from build123d import *
from build123d.topology import SkipClean

# Parameters (mm, degrees)
SKETCH1_W           = 30
SKETCH1_H           = 30
SKETCH1_W_2         = 2
SKETCH1_H_2         = 10
BOSS_EXTRUDE1_DEPTH = 75
SKETCH2_W           = 30
SKETCH2_H           = 22.5
CUT_EXTRUDE1_DEPTH  = 75
SKETCH3_W           = 26
SKETCH3_H           = 30.082215134
CUT_EXTRUDE2_DEPTH  = 28
SKETCH5_R           = 2.5
CUT_EXTRUDE3_DEPTH  = 38
BOSS_EXTRUDE2_DEPTH = 2
BOSS_EXTRUDE3_START = 2
BOSS_EXTRUDE3_DEPTH = 2
SKETCH9_R           = 2.5
CUT_EXTRUDE4_DEPTH  = 169.967145294


with BuildPart() as part:
    # Sketch1 → Boss-Extrude1 (new body)
    with BuildSketch(Plane.XY):
        Rectangle(SKETCH1_W, SKETCH1_H)
        with BuildLine():
            Line((50.917737084, -85.641756384), (53, -85.641756384))
            ThreePointArc((53, -85.641756384), (42.989370072, -49.687860894), (15, -25))
            Line((15, -25), (14.157929479, -26.814088542))
            ThreePointArc((14.157929479, -26.814088542), (41.246515654, -50.786104008), (50.917737084, -85.641756384))
        make_face()
        with Locations((14, -20)):
            Rectangle(SKETCH1_W_2, SKETCH1_H_2)
        Polygon((14.157929479, -26.814088542), (15, -25), (13, -25), (13, -26.814088542), align=None)
        with BuildLine():
            Line((12.135037198, -143.180046466), (13, -144.983332176))
            ThreePointArc((13, -144.983332176), (41.796634815, -121.242036174), (53, -85.641756384))
            Line((53, -85.641756384), (50.917737084, -85.641756384))
            ThreePointArc((50.917737084, -85.641756384), (40.047121172, -120.154156399), (12.135037198, -143.180046466))
        make_face()
    extrude(amount=BOSS_EXTRUDE1_DEPTH)

    # Sketch2 → Cut-Extrude1 (cut)
    with BuildSketch(Plane(origin=(0, 15, 0), x_dir=(1, 0, 0), z_dir=(0, 1, 0))):
        with Locations((0, -11.25)):
            Rectangle(SKETCH2_W, SKETCH2_H)
        with Locations((0, -63.75)):
            Rectangle(SKETCH2_W, SKETCH2_H)
    extrude(amount=-CUT_EXTRUDE1_DEPTH, mode=Mode.SUBTRACT)

    # Sketch3 → Cut-Extrude2 (cut)
    with BuildSketch(Plane.ZY.offset(15)):
        with Locations((37.5, 0.030332794)):
            Rectangle(SKETCH3_W, SKETCH3_H)
    extrude(amount=-CUT_EXTRUDE2_DEPTH, mode=Mode.SUBTRACT)

    # Sketch5 → Cut-Extrude3 (cut)
    with BuildSketch(Plane.XY.offset(52.5)):
        Circle(SKETCH5_R)
    extrude(amount=-CUT_EXTRUDE3_DEPTH, mode=Mode.SUBTRACT)

    # Sketch6 → Boss-Extrude2 (add)
    with SkipClean():  # the faces are left unmerged after this step: merging them gives an invalid solid
        with BuildSketch(Plane.XY.offset(75)):
            with BuildLine():
                Line((13, -144.983332176), (13, -94.983332176))
                Line((13, -94.983332176), (52.174379027, -94.983332176))
                ThreePointArc((52.174379027, -94.983332176), (39.036739849, -125.036474764), (13, -144.983332176))
            make_face()
        extrude(amount=BOSS_EXTRUDE2_DEPTH)

    # Sketch7 → Boss-Extrude3 (add)
    with SkipClean():  # the faces are left unmerged after this step: merging them gives an invalid solid
        with BuildSketch(Plane(origin=(0, 0, 0), x_dir=(-1, 0, 0), z_dir=(0, 0, -1)).offset(BOSS_EXTRUDE3_START)):
            with BuildLine():
                Line((-13, -144.983332176), (-13, -94.983332176))
                Line((-13, -94.983332176), (-52.174379027, -94.983332176))
                ThreePointArc((-52.174379027, -94.983332176), (-39.036739849, -125.036474764), (-13, -144.983332176))
            make_face()
        extrude(amount=-BOSS_EXTRUDE3_DEPTH)

    # Sketch9 → Cut-Extrude4 (cut, through all)
    with SkipClean():  # the faces are left unmerged after this step: merging them gives an invalid solid
        with BuildSketch(Plane.ZY.offset(-13)):
            with Locations((37.5, -61.814088542)):
                Circle(SKETCH9_R)
        extrude(amount=-CUT_EXTRUDE4_DEPTH, mode=Mode.SUBTRACT)


solid = part.part
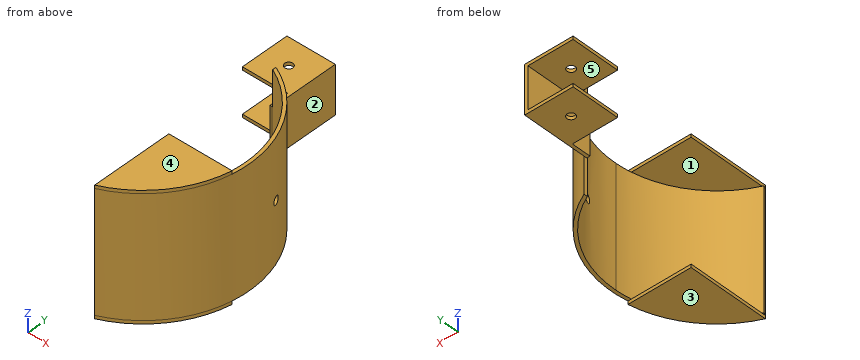
Can you work these out from the model? Positions are in its coordinate system, mm. Face numbers are marked on the shaded views. A direction names the side the tool comes from. Give positions to 0.01 mm unless a question says otherwise; leave off trailing zeros. Loops run counter-clockwise (first coordinate to the right, second up) from the corner with the lowest first, then second, coordinate; pieces in that order, holes last. Notation, with made-up numbers: (68, 40.5) -> (98, 40.5) arc R19 ccw to (98, 71.5) -> close; hole circle Ø2 at (-36, -12.5). An arc over 180 degrees is marked (long way). Return JSON: item names as keys, results as strings.
Q1. For pin 1 Ø2 at (x, z) = (-2.5, 51.5) entering from -Y; pin 2 Ø1 at (x, z) = (32, 76) entering from +Y; pin 3 Ø3 at (y, z) = (-80, 34.5) entering from -X, each with a flat end and sliding along its axis, tell me the tip position at first contact or that it passes through.
Checks:
{"pin 1": "stops at y = -15", "pin 2": "stops at y = -94.98", "pin 3": "stops at x = 50.64"}
Q2. I want a section at A-A, the plane x = 0. List the corners of the cut face in (y, z) for me, then the cut area to 3 significant figures.
Checks:
{"outline": "(-15, 22.5) -> (-2.5, 22.5) -> (-2.5, 24.5) -> (-15, 24.5) -> close; (-15, 50.5) -> (-2.5, 50.5) -> (-2.5, 52.5) -> (-15, 52.5) -> close; (2.5, 22.5) -> (15, 22.5) -> (15, 24.5) -> (2.5, 24.5) -> close; (2.5, 50.5) -> (15, 50.5) -> (15, 52.5) -> (2.5, 52.5) -> close", "area": "100 mm2"}
Q3. I need wall thicknesses on probe 1 along Y at (x, z) = (0, 51.55); probe 2 along Z at (x, y) = (-9.5, -9); probe 3 along X at (y, z) = (-12.5, 44). Which ranges of each line are inside material? Lowest first, please.
Checks:
{"probe 1": "y = -15 to -2.5, 2.5 to 15", "probe 2": "z = 22.5 to 24.5, 50.5 to 52.5", "probe 3": "x = 13 to 15"}
Q4. On a 3-axis mill with a long thin cutter (end or side, diameter ignored), from which of +Z, -Z, +X, -X, +Y, -Y can I reach the whole of each face in a straight line? I mean the marked faces 1 and 2. Say none if no direction works.
Checks:
{"face 1": "-X", "face 2": "+Z, -Z, +X, +Y"}
Q5. I want a section at D-D, the plane z = 7. List the corners of the cut face in (x, y) for me, then the cut area to 3 significant figures.
Checks:
{"outline": "(12.14, -143.18) -> (13, -144.98) arc R65.65 ccw to (15, -25) -> (15, -27.21) arc R63.71 cw to start", "area": "305 mm2"}
Q6. We'd pull the mould along Z, two halves only. Please class the marked faces 3, 4 and 5: released by +Z, released by -Z, zero draft, split by the parting line, or undercut.
Checks:
{"face 3": "released by -Z", "face 4": "released by +Z", "face 5": "undercut"}
Q7. I want a section at B-B, the plane y = 0. List the corners of the cut face in (x, z) for me.
Checks:
{"outline": "(-15, 22.5) -> (-2.5, 22.5) -> (-2.5, 24.5) -> (-15, 24.5) -> close; (-15, 50.5) -> (-2.5, 50.5) -> (-2.5, 52.5) -> (-15, 52.5) -> close; (2.5, 22.5) -> (15, 22.5) -> (15, 52.5) -> (2.5, 52.5) -> (2.5, 50.5) -> (13, 50.5) -> (13, 24.5) -> (2.5, 24.5) -> close"}
Q8. I want a section at C-C, the plane z = 37.5. List the corners of the cut face in (x, y) for me, then the cut area to 3 significant figures.
Checks:
{"outline": "(12.14, -143.18) -> (13, -144.98) arc R65.65 ccw to (49.81, -64.31) -> (47.63, -64.31) arc R63.71 cw to start; (13, -26.81) -> (14.16, -26.81) arc R63.71 cw to (45.72, -59.31) -> (47.97, -59.31) arc R65.65 ccw to (15, -25) -> (15, 15) -> (13, 15) -> close", "area": "378 mm2"}
